Check sheet for the modelled part. Datum: model origin and axes. Units: mm. A direction names the side the tool comes from. Round coordinates to 2 decimals unless told otherwise and drop trailing zeros. Loops run counter-clockwise (first coordinate to the right, second up) from the corner with the lowest first, then second, coordinate; pieces in that order, holes last. Notation, with made-up numbers: (-27, 21.5) -> (-6, 21.5) arc R20 cw to (-6, 39.5) -> close; hole circle Ø6 at (-0.75, -33.75). An arc over 180 degrees is marked (long way). Return JSON: item names as keys, results as strings.
from build123d import *

# Parameters (mm, degrees)
SKETCH1_R           = 12.5
SKETCH1_R_2         = 5.1
BOSS_EXTRUDE1_DEPTH = 20
SKETCH2_R           = 5.1
SKETCH2_R_2         = 2.6
BOSS_EXTRUDE2_DEPTH = 10
CUT_EXTRUDE1_REACH  = 14.5
SKETCH3_R           = 1.8
CHAMFER1_SIZE       = 0.75


with BuildPart() as part:
    # Sketch1 → Boss-Extrude1 (new body)
    with BuildSketch(Plane(origin=(0, 0, 0), x_dir=(0, 0, -1), z_dir=(1, 0, 0))):
        Circle(SKETCH1_R)
        Circle(SKETCH1_R_2, mode=Mode.SUBTRACT)
    extrude(amount=BOSS_EXTRUDE1_DEPTH)

    # Sketch2 → Boss-Extrude2 (add)
    with BuildSketch(Plane(origin=(20, 0, 0), x_dir=(0, 0, -1), z_dir=(1, 0, 0))):
        Circle(SKETCH2_R)
        Circle(SKETCH2_R_2, mode=Mode.SUBTRACT)
    extrude(amount=-BOSS_EXTRUDE2_DEPTH)

    # Sketch3 → Cut-Extrude1 (cut, up to next)
    with BuildSketch(Plane(origin=(0, 0, 0), x_dir=(1, 0, 0), z_dir=(0, 1, 0)), mode=Mode.PRIVATE) as cut_extrude1_sk1:
        with Locations((5, 0)):
            Circle(SKETCH3_R)
    cut_extrude1_tool1 = extrude(cut_extrude1_sk1.sketch, amount=CUT_EXTRUDE1_REACH, mode=Mode.PRIVATE) & part.part
    add(cut_extrude1_tool1.solids().sort_by_distance((5, 0, 0))[0], mode=Mode.SUBTRACT)
    # Sketch3 → Cut-Extrude1 (cut, up to next)
    with BuildSketch(Plane(origin=(0, 0, 0), x_dir=(1, 0, 0), z_dir=(0, 1, 0)), mode=Mode.PRIVATE) as cut_extrude1_sk2:
        with Locations((15, 0)):
            Circle(SKETCH3_R)
    cut_extrude1_tool2 = extrude(cut_extrude1_sk2.sketch, amount=CUT_EXTRUDE1_REACH, mode=Mode.PRIVATE) & part.part
    add(cut_extrude1_tool2.solids().sort_by_distance((15, 0, 0))[0], mode=Mode.SUBTRACT)

    # Chamfer1
    chamfer1_edges = [part.edges().sort_by_distance(p)[0] for p in [
        (10, 0, 5.1),
        (20, 0, 2.6),
        (0, 0, 12.5),
        (20, 0, 12.5),
        (0, 0, 5.1),
    ]]
    chamfer(chamfer1_edges, length=CHAMFER1_SIZE)


solid = part.part
Q1. Draft check along Y on faces 1 (the cylindrical face through (4.9, -4.5, -2.4)), 2 (the cylindrical face through (9.87, -11.09, -5.77)), 3 (the cylindrical face through (13.2, 7.12, -0.08)). Enter one of: released by +Y, released by -Y, zero draft, split by the parting line, or undercut.
Results list:
{"face 1": "undercut", "face 2": "split by the parting line", "face 3": "zero draft"}
Q2. Material ranges on line 1 (X direction, y = 9, z = 0); line 2 (Z direction, x = 5, y = 9.25); line 3 (X direction, y = -10.75, z = -4.75), recorded low to high.
Results list:
{"line 1": "0 to 3.2, 6.8 to 13.2, 16.8 to 20", "line 2": "-8.41 to -1.8, 1.8 to 8.41", "line 3": "0 to 20"}
Q3. Section check B-B (z = 0). Count the separate pieces of the cut face and the enclosed holes in it, then the cut area to 3 significant figures.
Results list:
{"separate pieces": "4", "enclosed holes": "0", "area": "282 mm^2"}
Q4. Go/stop test with flat-tipped pins: pin 1 (1.5 mm diameter, centred on x = 17, y = -2, fed in from +Z); pin 2 (4 mm diameter, centred on x = 3, z = -7.5, fed in from +Y) (3 decimals); pin 3 (4.5 mm diameter, centred on y = -1.5, z = 2, fed in from -X); pin 4 (3 mm diameter, centred on y = 0, z = 0, fed in from -X). Record where each tip stops, or that it passes through.
Results list:
{"pin 1": "z = 12.44", "pin 2": "y = 11.225", "pin 3": "x = 9.6", "pin 4": "through"}
Q5. Tool access check on faces 4 (the cylindrical face through (6.717, 8.583, -0.541)), 5 (the flat face through (10, -2, -2)), 6 (the flat face through (0, 2.8, 5.4)). Record the directions out of +Z, -Z, +X, -X, +Y, -Y that give a thin tool (end or side, any length) a straight path to the whole face; none if there is none.
Results list:
{"face 4": "+Y", "face 5": "-X", "face 6": "+Z, -Z, -X, +Y, -Y"}
Q6. Section check C-C (x = 7.25). Record the boundary of the cut face in (y, z), then the cut area to 3 significant figures.
Results list:
{"outline": "circle Ø25 at (0, 0); hole circle Ø10.2 at (0, 0)", "area": "409 mm^2"}
Q7. Section check A-A (y = 0). Record the boundary of the cut face in (x, z).
Results list:
{"outline": "(0, -11.75) -> (0.75, -12.5) -> (19.25, -12.5) -> (20, -11.75) -> (20, -3.35) -> (19.25, -2.6) -> (10, -2.6) -> (10, -4.35) -> (9.25, -5.1) -> (0.75, -5.1) -> (0, -5.85) -> close; (0, 5.85) -> (0.75, 5.1) -> (9.25, 5.1) -> (10, 4.35) -> (10, 2.6) -> (19.25, 2.6) -> (20, 3.35) -> (20, 11.75) -> (19.25, 12.5) -> (0.75, 12.5) -> (0, 11.75) -> close"}
